```python
from build123d import *

# Parameters (mm, degrees)
SKETCH1_R           = 1.5
BOSS_EXTRUDE1_DEPTH = 5
SKETCH1_3_W         = 10
SKETCH1_3_H         = 24
CUT_EXTRUDE1_DEPTH  = 6
SKETCH1_4_W         = 5
SKETCH1_4_H         = 42
BOSS_EXTRUDE2_DEPTH = 42
BOSS_EXTRUDE3_DEPTH = 21
SKETCH4_W           = 24
SKETCH4_H           = 5
CUT_EXTRUDE2_DEPTH  = 6
SKETCH5_R           = 0.99
BOSS_EXTRUDE4_DEPTH = 5


with BuildPart() as part:
    # Sketch1 → Boss-Extrude1 (new body)
    with BuildSketch(Plane(origin=(0, 0, 0), x_dir=(1, 0, 0), z_dir=(0, 1, 0))):
        Polygon((-44.5, -32), (44.5, -32), (44.5, -12), (44.5, 12), (44.5, 32), (-44.5, 32), align=None)
        with Locations((-42.25, -30)):
            Circle(SKETCH1_R, mode=Mode.SUBTRACT)
        with Locations((42.25, -29.5)):
            Circle(SKETCH1_R, mode=Mode.SUBTRACT)
        with Locations((-42.25, 30)):
            Circle(SKETCH1_R, mode=Mode.SUBTRACT)
        with Locations((42.25, 29.5)):
            Circle(SKETCH1_R, mode=Mode.SUBTRACT)
    extrude(amount=BOSS_EXTRUDE1_DEPTH)

    # Sketch1<3> → Cut-Extrude1 (cut, through all)
    with BuildSketch(Plane(origin=(0, 0, 0), x_dir=(1, 0, 0), z_dir=(0, 1, 0))):
        with Locations((29.5, 0)):
            Rectangle(SKETCH1_3_W, SKETCH1_3_H)
    extrude(amount=CUT_EXTRUDE1_DEPTH, mode=Mode.SUBTRACT)

    # Sketch1<4> → Boss-Extrude2 (add)
    with BuildSketch(Plane(origin=(0, 0, 0), x_dir=(1, 0, 0), z_dir=(0, 1, 0))):
        with Locations((16, 0)):
            Rectangle(SKETCH1_4_W, SKETCH1_4_H)
    extrude(amount=BOSS_EXTRUDE2_DEPTH)

    # Sketch3 → Boss-Extrude3 (add, symmetric)
    with BuildSketch(Plane.XY):
        Polygon((13.5, 23.5), (0, 5), (13.5, 5), align=None)
    extrude(amount=BOSS_EXTRUDE3_DEPTH, both=True)

    # Sketch4 → Cut-Extrude2 (cut)
    with BuildSketch(Plane(origin=(24.5, 0, 0), x_dir=(0, 0, -1), z_dir=(1, 0, 0))):
        with Locations((0, 2.5)):
            Rectangle(SKETCH4_W, SKETCH4_H)
    extrude(amount=-CUT_EXTRUDE2_DEPTH, mode=Mode.SUBTRACT)

    # Sketch5 → Boss-Extrude4 (add)
    with BuildSketch(Plane(origin=(18.5, 0, 0), x_dir=(0, 0, -1), z_dir=(1, 0, 0))):
        with Locations((-10.5, 37)):
            Circle(SKETCH5_R)
        with Locations((10.5, 37)):
            Circle(SKETCH5_R)
        with Locations((10.5, 24.5)):
            Circle(SKETCH5_R)
        with Locations((-10.5, 24.5)):
            Circle(SKETCH5_R)
    extrude(amount=BOSS_EXTRUDE4_DEPTH)


solid = part.part
```
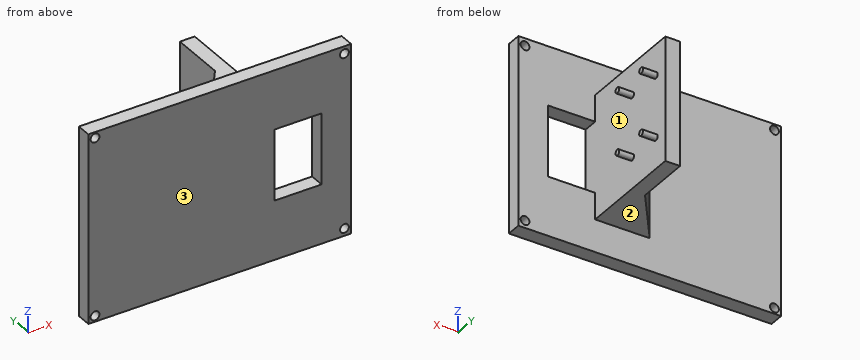
Geometry: final body of the model. Coordinates: model frame, mm. Face numbers are marked on the shaded views. Coordinates: 2 decimals unless noted, no trailing zeros. Write each loop counter-clockwise with the first axis right and the second up, starting at its lowest first coordinate (ties: lowest second). Pieces come first, ordered by that corner, then holes. Notation, with made-up numbers: M 49.25,-7.5 L 55.25,-7.5 A15 ccw 55.25,-1.5 Z; hole C 49.5,-14 d8. An arc over 180 degrees is marked long. Use CSV: the item, a comma, the result in double quotes. Start each with the question number.
1. First-contact query: P1, Ø1.8, axis at x = 42.25, z = 29.5, coming from the +Y side; P2, Ø8, axis at x = 14.5, y = 21.5, coming from the -Z side; P3, Ø1, axis at y = 37.5, z = 11, coming from the +X side; P4, Ø5, axis at y = 23, z = 21, coming from the -X side. Flat tips, straight axial feed; report the tip coordinate or a pass-through.
2. Cut plane A-A on z = 2.5. Return the cut outline in (x, y).
3. Cut plane C-C on x = 21. Return the cut outline in (y, z), plus the area to 3 significant figures.
4. Ray query, probe 1 along Z at (x, y) = (42, 2); probe 2 along Z at (x, y) = (-42, 3); probe 3 along X at (y, z) = (2.7, -30). Return the intervals inside material, ascending.
5. Cut plane D-D on z = 14.5. Return the cut outline in (x, y).
6. Mould query, pull axis Z, two halves, no side actions, for the marked faces 1, 2 and 3. Classes: pulls with the +Z half, pulls with the -Z half, needs draft (parallel to the pull), parting line crosses it, or undercut.
7. Cut plane B-B on x = 31. Return the cut outline in (y, z).
Entries:
1,P1,"through"
1,P2,"z = -21"
1,P3,"x = 23.5"
1,P4,"x = 11.31"
2,outline,"M -44.5,0 L 18.5,0 L 18.5,42 L 13.5,42 L 13.5,23.5 L 0,5 L -44.5,5 Z; M 34.5,0 L 44.5,0 L 44.5,5 L 34.5,5 Z"
3,outline,"M 0,-32 L 5,-32 L 5,-12 L 0,-12 Z; M 0,12 L 5,12 L 5,32 L 0,32 Z; C 24.5,-10.5 d1.98; C 24.5,10.5 d1.98; C 37,-10.5 d1.98; C 37,10.5 d1.98"
3,area,"212 mm²"
4,probe 1,"-32 to -30.98, -28.02 to 28.02, 30.98 to 32"
4,probe 2,"-32 to -31.48, -28.52 to 28.52, 31.48 to 32"
4,probe 3,"-44.5 to -43.75, -40.75 to 40.84, 43.66 to 44.5"
5,outline,"M -44.5,0 L 44.5,0 L 44.5,5 L 18.5,5 L 18.5,42 L 13.5,42 L 13.5,23.5 L 0,5 L -44.5,5 Z"
6,face 1,"undercut"
6,face 2,"pulls with the -Z half"
6,face 3,"needs draft"
7,outline,"M 0,-32 L 5,-32 L 5,-12 L 0,-12 Z; M 0,12 L 5,12 L 5,32 L 0,32 Z"
